Design review of the part built by this model. Coordinates are the model's own, in mm. A direction names the side the tool comes from. Coordinates: 2 decimals unless noted, no trailing zeros. Use a Markdown table: item, result.
Solid Edge part; units mm, degrees
sketch "Sketch1" plane through (0, 0, 0) normal (0, 0, 1) x (1, 0, 0)
  line L0 (88.8945, 25.9382) -> (88.8945, 40.9382)
  line L1 (-11.6502, 40.9382) -> (88.8945, 40.9382)
  line L2 (-11.6502, -39.0633) -> (-11.6502, 40.9382)
  line L3 (88.8945, -39.0633) -> (-11.6502, -39.0633)
  line L4 (88.8945, -39.0633) -> (88.8945, -24.0633)
  line L5 (88.8945, 25.9382) -> (88.8945, -24.0633)
  circle A0 centre (38.6222, 30.8554) radius 2
  circle A1 centre (38.6222, -29.0633) radius 2
  circle A2 centre (-0.7269, 30.8554) radius 2
  circle A3 centre (-0.2702, 0.8589) radius 2
  circle A4 centre (0.1865, -29.1376) radius 2
  circle A5 centre (77.8945, -29.0633) radius 2
  circle A6 centre (77.8945, 0.9299) radius 2
  circle A7 centre (77.8945, 30.9382) radius 2
extrude "Protrusion1" add sketch "Sketch1" along normal blind 3
sketch "Sketch2" plane through (38.6222, 0.9374, 3) normal (0, 0, 1) x (1, 0, 0)
  line L0 (-44.3491, 24.918) -> (-34.3491, 24.918)
  line L1 (-34.3491, 24.918) -> (-34.3491, 34.918)
  line L2 (-34.3491, 34.918) -> (-44.3491, 34.918)
  line L3 (-44.3491, 34.918) -> (-44.3491, 24.918)
  line L4 (34.2724, 25.0007) -> (44.2724, 25.0007)
  line L5 (44.2724, 25.0007) -> (44.2724, 35.0007)
  line L6 (44.2724, 35.0007) -> (34.2724, 35.0007)
  line L7 (34.2724, 35.0007) -> (34.2724, 25.0007)
  line L8 (34.2724, -5.0076) -> (44.2724, -5.0076)
  line L9 (44.2724, -5.0076) -> (44.2724, 4.9924)
  line L10 (44.2724, 4.9924) -> (34.2724, 4.9924)
  line L11 (34.2724, 4.9924) -> (34.2724, -5.0076)
  line L12 (34.2724, -35.0007) -> (44.2724, -35.0007)
  line L13 (44.2724, -35.0007) -> (44.2724, -25.0007)
  line L14 (44.2724, -25.0007) -> (34.2724, -25.0007)
  line L15 (34.2724, -25.0007) -> (34.2724, -35.0007)
  line L16 (-43.4356, -35.0751) -> (-33.4356, -35.0751)
  line L17 (-33.4356, -35.0751) -> (-33.4356, -25.0751)
  line L18 (-33.4356, -25.0751) -> (-43.4356, -25.0751)
  line L19 (-43.4356, -25.0751) -> (-43.4356, -35.0751)
  line L20 (-43.8924, -5.0785) -> (-33.8924, -5.0785)
  line L21 (-33.8924, -5.0785) -> (-33.8924, 4.9215)
  line L22 (-33.8924, 4.9215) -> (-43.8924, 4.9215)
  line L23 (-43.8924, 4.9215) -> (-43.8924, -5.0785)
extrude "ExtrudedCutout_1" cut sketch "Sketch2" against normal blind 1.5
sketch "Sketch3" plane through (38.6222, 0.9374, 0) normal (0, 0, -1) x (1, 0, 0)
  line L0 (-45.4356, 26.0336) -> (-38.4356, 21.9922)
  line L1 (-38.4356, 21.9922) -> (-31.4356, 26.0336)
  line L2 (-31.4356, 26.0336) -> (-31.4356, 34.1165)
  line L3 (-31.4356, 34.1165) -> (-38.4356, 38.158)
  line L4 (-38.4356, 38.158) -> (-45.4356, 34.1165)
  line L5 (-45.4356, 34.1165) -> (-45.4356, 26.0336)
  line L6 (-45.8924, -3.9629) -> (-38.8924, -8.0044)
  line L7 (-38.8924, -8.0044) -> (-31.8924, -3.9629)
  line L8 (-31.8924, -3.9629) -> (-31.8924, 4.12)
  line L9 (-31.8924, 4.12) -> (-38.8924, 8.1614)
  line L10 (-38.8924, 8.1614) -> (-45.8924, 4.12)
  line L11 (-45.8924, 4.12) -> (-45.8924, -3.9629)
  line L12 (-32.3491, -25.8765) -> (-39.3491, -21.8351)
  line L13 (-39.3491, -21.8351) -> (-46.3491, -25.8765)
  line L14 (-46.3491, -25.8765) -> (-46.3491, -33.9594)
  line L15 (-46.3491, -33.9594) -> (-39.3491, -38.0009)
  line L16 (-39.3491, -38.0009) -> (-32.3491, -33.9594)
  line L17 (-32.3491, -33.9594) -> (-32.3491, -25.8765)
  line L18 (7, -25.8765) -> (0, -21.8351)
  line L19 (0, -21.8351) -> (-7, -25.8765)
  line L20 (-7, -25.8765) -> (-7, -33.9594)
  line L21 (-7, -33.9594) -> (0, -38.0009)
  line L22 (0, -38.0009) -> (7, -33.9594)
  line L23 (7, -33.9594) -> (7, -25.8765)
  line L24 (7, 34.0422) -> (0, 38.0836)
  line L25 (0, 38.0836) -> (-7, 34.0422)
  line L26 (-7, 34.0422) -> (-7, 25.9593)
  line L27 (-7, 25.9593) -> (0, 21.9178)
  line L28 (0, 21.9178) -> (7, 25.9593)
  line L29 (7, 25.9593) -> (7, 34.0422)
  line L30 (46.2724, 4.049) -> (39.2724, 8.0905)
  line L31 (39.2724, 8.0905) -> (32.2724, 4.049)
  line L32 (32.2724, 4.049) -> (32.2724, -4.0339)
  line L33 (32.2724, -4.0339) -> (39.2724, -8.0753)
  line L34 (39.2724, -8.0753) -> (46.2724, -4.0339)
  line L35 (46.2724, -4.0339) -> (46.2724, 4.049)
  line L36 (46.2724, 34.0422) -> (39.2724, 38.0836)
  line L37 (39.2724, 38.0836) -> (32.2724, 34.0422)
  line L38 (32.2724, 34.0422) -> (32.2724, 25.9593)
  line L39 (32.2724, 25.9593) -> (39.2724, 21.9178)
  line L40 (39.2724, 21.9178) -> (46.2724, 25.9593)
  line L41 (46.2724, 25.9593) -> (46.2724, 34.0422)
  line L42 (46.2724, -25.9593) -> (39.2724, -21.9178)
  line L43 (39.2724, -21.9178) -> (32.2724, -25.9593)
  line L44 (32.2724, -25.9593) -> (32.2724, -34.0422)
  line L45 (32.2724, -34.0422) -> (39.2724, -38.0836)
  line L46 (39.2724, -38.0836) -> (46.2724, -34.0422)
  line L47 (46.2724, -34.0422) -> (46.2724, -25.9593)
  line L48 (-50.2724, 40.0007) -> (50.2724, 40.0007)
  line L49 (50.2724, 40.0007) -> (50.2724, -40.0007)
  line L50 (50.2724, -40.0007) -> (-50.2724, -40.0007)
  line L51 (-50.2724, -40.0007) -> (-50.2724, 40.0007)
extrude "ExtrudedProtrusion_2" add sketch "Sketch3" along normal blind 1.5
(1) Draft analysis for pull direction Y (two halves, no side actions). For faces 3 (the flat face through (38, 1, -1.5)), 4 (the flat face through (42.17, 24.82, -0.74)), 5 (the flat face through (39, -39.063, 1)), state which applies: +Y half, -Y half, draft (parallel to the pull), parting line (faces both ways), or undercut.
Determined:
| item | result |
|---|---|
| face 3 | draft |
| face 4 | undercut |
| face 5 | -Y half |
(2) For pin 1 (7 mm diameter, centred on x = 76, y = 33.5, fed in from -Z); pin 2 (3 mm diameter, centred on x = -2, y = -31.5, fed in from +Z), all flat-tipped, find the tip position at first contact; note any pin that passes through.
Determined:
| item | result |
|---|---|
| pin 1 | z = 0 |
| pin 2 | z = 1.5 |
(3) Machinability: for faces 1 (the cylindrical face through (40.47, 31.62, 1.48)), 2 (the flat face through (74.346, -23.029, -0.74)), which of the approach directions +Z, -Z, +X, -X, +Y, -Y give a long, thin tool a straight path to every point of the face, cutting with its end or side? Answer none if there is none.
Determined:
| item | result |
|---|---|
| face 1 | +Z, -Z |
| face 2 | -Z |
(4) Take a section at A-A on z = 2.2. State how many separate pieces and enclosed holes the cut face has, and give its area (3 significant figures).
Determined:
| item | result |
|---|---|
| separate pieces | 1 |
| enclosed holes | 8 |
| area | 7,420 mm2 |
(5) For L1, parallel to Y at x = 76, z = 2.5; L2, parallel to X at y = 3.5, z = 2.1; L3, parallel to X at y = 1, z = 0.6, list the stretches that pass through material, from the lowest coordinate up. Write a range as from..to.
Determined:
| item | result |
|---|---|
| L1 | -39.06..-34.06, -24.06..-4.07, 5.93..25.94, 35.94..40.94 |
| L2 | -11.65..-5.27, 4.73..72.89, 82.89..88.89 |
| L3 | -11.65..-2.27, 1.72..75.9, 79.89..88.89 |
